For this review, take the finished solid that the model builds, in its own axes (mm). Round coordinates to 2 decimals unless told otherwise and drop trailing zeros. Write each loop counter-clockwise with the first axis right and the second up, starting at its lowest first coordinate (ties: lowest second). Pieces come first, ordered by that corner, then holes.
from build123d import *

# Parameters (mm, degrees)
SKETCH1_R           = 8.371232018
BOSS_EXTRUDE1_DEPTH = 10
FILLET1_R           = 5


with BuildPart() as part:
    # Sketch1 → Boss-Extrude1 (new body)
    with BuildSketch(Plane(origin=(0, 0, 0), x_dir=(0, 0, -1), z_dir=(1, 0, 0))):
        with BuildLine():
            Line((46.963546465, -11.666577207), (-46.963546465, -11.666577207))
            Line((-46.963546465, -11.666577207), (-46.963546465, 0))
            add(Edge.make_bspline(
                [(-46.963546465, 0), (-16.221096815, 9.567463223), (-14.267406521, 43.471004243)],
                knots=[0, 0, 0, 1, 1, 1], degree=2))
            ThreePointArc((-14.267406521, 43.471004243), (0, 57.738410764), (14.267406521, 43.471004243))
            add(Edge.make_bspline(
                [(46.963546465, 0), (16.221096815, 9.567463223), (14.267406521, 43.471004243)],
                knots=[0, 0, 0, 1, 1, 1], degree=2))
            Line((46.963546465, 0), (46.963546465, -11.666577207))
        make_face()
        with Locations((0, 43.471004243)):
            Circle(SKETCH1_R, mode=Mode.SUBTRACT)
    extrude(amount=BOSS_EXTRUDE1_DEPTH)

    # Fillet1
    fillet1_edges = [part.edges().sort_by_distance(p)[0] for p in [
        (5, 0, 46.963546465),
        (5, 0, -46.963546465),
    ]]
    fillet(fillet1_edges, radius=FILLET1_R)


solid = part.part
(1) We need section A-A, the plane z = 0. Give the boundary of the cut face in (x, y), and give its area (3 significant figures).
Geometry check:
outline: (0, -11.67) - (10, -11.67) - (10, 35.1) - (0, 35.1) - close; (0, 51.84) - (10, 51.84) - (10, 57.74) - (0, 57.74) - close
area: 527 mm2
(2) Mouldability with a two-part tool opening along Z and no side actions: class faces 1 (the face through (4.93, 57.735, 0.314)), 2 (the face through (5, -11.667, -1)), 3 (the face through (4.93, 51.77, 1.09)) as pulls with the +Z half, pulls with the -Z half, needs draft (parallel to the pull), parting line crosses it, or undercut.
Geometry check:
face 1: parting line crosses it
face 2: needs draft
face 3: undercut
(3) For pin 1 Ø1.5 at (x, y) = (1.5, 42.5) entering from -Z; pin 2 Ø4 at (x, z) = (7.5, -3.5) entering from +Y; pin 3 Ø3 at (x, y) = (6, 44) entering from -Z; pin 4 Ø12 at (y, z) = (8, 8) entering from -X, all flat-tipped, find the tip position at first contact; note any pin that passes through.
Geometry check:
pin 1: stops at z = -14.39
pin 2: stops at y = 57.66
pin 3: stops at z = -14.33
pin 4: stops at x = 0
(4) For line 1 along Z through (x, y) = (9.5, 44); line 2 along Y through (x, z) = (6, 0); line 3 along Z through (x, y) = (6, 38), list the stretches that pass through material, from the lowest coordinate up.
Geometry check:
line 1: z = -14.26 to -8.35, 8.35 to 14.26
line 2: y = -11.67 to 35.1, 51.84 to 57.74
line 3: z = -14.79 to -6.34, 6.34 to 14.79
